Read the model definition and answer for the solid it produces. Units are mm, in the model's axes. A direction names the side the tool comes from. Round coordinates to 2 decimals unless told otherwise and drop trailing zeros. Order: outer loops, then holes, each group sorted by start corner. A loop starts at its lowest first (then second) coordinate and runs counter-clockwise, first axis right, second up. Notation, with made-up numbers: (-15, 56.25) - (24, 56.25) arc R17 cw to (24, 72.25) - close; hole circle Ø1 at (6, 22). An arc over 180 degrees is marked (long way). Answer as a JSON object with one key per item and string values. Group by question number.
Q1. A cutting plane is placed at A-A on y = 0. Determine the outline of the cut face in (x, z).
Q2. Given pin 1 Ø1 at (x, y) = (-5, -6) entering from +Z; pin 2 Ø1.5 at (y, z) = (-11.5, 0.5) entering from -X; pin 3 Ø8 at (x, y) = (-12.5, 7.5) entering from -Z; pin 4 Ø2 at (x, z) = (-24, 3.5) entering from +Y, each flat-ended and moving along its own axis, determine where each tip first touches the part or whether it passes through.
Q3. A tool of negligible diameter and unlimited length cuts with its end or side. For faces 5 (the flat face through (33.865, 16.365, 2.958)), 6 (the cylindrical face through (36.963, 15.287, 2.958)), 7 (the flat face through (24.6, 28.54, 2.96)), 8 (the flat face through (-28.476, -24.572, 2.958)), 9 (the flat face through (-31.105, 21.146, 2.958)), from which of +Z, -Z, +X, -X, +Y, -Y can it reach the whole face along a straight path? Write none if from no direction.
Q4. Consider line 1 (X direction, y = 32, z = 1.5); line 2 (X direction, y = 36, z = 0.75); line 3 (X direction, y = 18, z = 4.8). Determine where each line is inside the solid, lowest interval first.
Q5. The mould has two halves that part along Y. Classify faces 1 (the cylindrical face through (-36.963, -15.287, 2.958)), 2 (the flat face through (-24.572, 28.476, 2.958)), 3 (the flat face through (2.76, 37.51, 2.96)), 4 (the flat face through (16.365, -33.865, 2.958)): pulls with the +Y half, pulls with the -Y half, needs draft (parallel to the pull), parting line crosses it, or undercut.
```python
from build123d import *

# Parameters (mm, degrees)
SKETCH1_R           = 40
SKETCH1_R_2         = 10
BOSS_EXTRUDE1_DEPTH = 6
CUT_EXTRUDE1_START  = -6
CUT_EXTRUDE1_DEPTH  = 6
CIRPATTERN1_DEPTH   = 6


# Read off the part's stored shape, not the designer's step: CirPattern1
with BuildPart() as part:
    # Sketch1 → Boss-Extrude1 (new body)
    with BuildSketch(Plane.XY):
        Circle(SKETCH1_R)
        Circle(SKETCH1_R_2, mode=Mode.SUBTRACT)
    extrude(amount=BOSS_EXTRUDE1_DEPTH)

    # Sketch2 → Cut-Extrude1 (cut)
    with BuildSketch(Plane.XY.offset(6).offset(CUT_EXTRUDE1_START)):
        with BuildLine():
            Line((-3.690328017, 39.829404705), (-1.856322788, 35.255644098))
            ThreePointArc((-1.856322788, 35.255644098), (0, 34), (1.856322788, 35.255644098))
            Line((1.856322788, 35.255644098), (3.690328017, 39.829404705))
            ThreePointArc((3.690328017, 39.829404705), (0, 40), (-3.690328017, 39.829404705))
        make_face()
    extrude(amount=CUT_EXTRUDE1_DEPTH, mode=Mode.SUBTRACT)

    # CirPattern1 outline → CirPattern1 (cut)
    with BuildSketch(Plane.XY):
        with BuildLine():
            ThreePointArc((-10.917902263, 33.573885466), (-8.799847534, 32.841478094), (-7.331762018, 34.534788848))
            Line((-7.331762018, 34.534788848), (-6.744025354, 39.427377824))
            ThreePointArc((-6.744025354, 39.427377824), (-10.352761804, 38.637033052), (-13.873191632, 37.517123477))
            Line((-13.873191632, 37.517123477), (-10.917902263, 33.573885466))
        make_face()
        with BuildLine():
            Line((10.917902263, 33.573885466), (13.873191632, 37.517123477))
            ThreePointArc((13.873191632, 37.517123477), (10.352761804, 38.637033052), (6.744025354, 39.427377824))
            Line((6.744025354, 39.427377824), (7.331762018, 34.534788848))
            ThreePointArc((7.331762018, 34.534788848), (8.799847534, 32.841478094), (10.917902263, 33.573885466))
        make_face()
        with BuildLine():
            Line((19.235444741, 29.604122022), (23.110620163, 32.648112284))
            ThreePointArc((23.110620163, 32.648112284), (20, 34.641016152), (16.718784541, 36.338440301))
            Line((16.718784541, 36.338440301), (16.020199358, 31.46044481))
            ThreePointArc((16.020199358, 31.46044481), (17, 29.444863729), (19.235444741, 29.604122022))
        make_face()
        with BuildLine():
            Line((26.242123448, 23.616886586), (30.773098123, 25.554186192))
            ThreePointArc((30.773098123, 25.554186192), (28.284271248, 28.284271248), (25.554186192, 30.773098123))
            Line((25.554186192, 30.773098123), (23.616886586, 26.242123448))
            ThreePointArc((23.616886586, 26.242123448), (24.04163056, 24.04163056), (26.242123448, 23.616886586))
        make_face()
        with BuildLine():
            Line((31.46044481, 16.020199358), (36.338440301, 16.718784541))
            ThreePointArc((36.338440301, 16.718784541), (34.641016152, 20), (32.648112284, 23.110620163))
            Line((32.648112284, 23.110620163), (29.604122022, 19.235444741))
            ThreePointArc((29.604122022, 19.235444741), (29.444863729, 17), (31.46044481, 16.020199358))
        make_face()
        with BuildLine():
            Line((34.534788848, 7.331762018), (39.427377824, 6.744025354))
            ThreePointArc((39.427377824, 6.744025354), (38.637033052, 10.352761804), (37.517123477, 13.873191632))
            Line((37.517123477, 13.873191632), (33.573885466, 10.917902263))
            ThreePointArc((33.573885466, 10.917902263), (32.841478094, 8.799847534), (34.534788848, 7.331762018))
        make_face()
        with BuildLine():
            Line((35.255644098, -1.856322788), (39.829404705, -3.690328017))
            ThreePointArc((39.829404705, -3.690328017), (40, 0), (39.829404705, 3.690328017))
            Line((39.829404705, 3.690328017), (35.255644098, 1.856322788))
            ThreePointArc((35.255644098, 1.856322788), (34, 0), (35.255644098, -1.856322788))
        make_face()
        with BuildLine():
            Line((33.573885466, -10.917902263), (37.517123477, -13.873191632))
            ThreePointArc((37.517123477, -13.873191632), (38.637033052, -10.352761804), (39.427377823, -6.744025354))
            Line((39.427377823, -6.744025354), (34.534788848, -7.331762018))
            ThreePointArc((34.534788848, -7.331762018), (32.841478094, -8.799847534), (33.573885466, -10.917902263))
        make_face()
        with BuildLine():
            Line((29.604122022, -19.235444741), (32.648112283, -23.110620163))
            ThreePointArc((32.648112283, -23.110620163), (34.641016152, -20), (36.3384403, -16.718784541))
            Line((36.3384403, -16.718784541), (31.46044481, -16.020199358))
            ThreePointArc((31.46044481, -16.020199358), (29.444863729, -17), (29.604122022, -19.235444741))
        make_face()
        with BuildLine():
            Line((23.616886586, -26.242123448), (25.554186192, -30.773098123))
            ThreePointArc((25.554186192, -30.773098123), (28.284271247, -28.284271247), (30.773098123, -25.554186192))
            Line((30.773098123, -25.554186192), (26.242123448, -23.616886586))
            ThreePointArc((26.242123448, -23.616886586), (24.04163056, -24.04163056), (23.616886586, -26.242123448))
        make_face()
        with BuildLine():
            Line((16.020199358, -31.46044481), (16.718784541, -36.3384403))
            ThreePointArc((16.718784541, -36.3384403), (20, -34.641016151), (23.110620163, -32.648112283))
            Line((23.110620163, -32.648112283), (19.235444741, -29.604122022))
            ThreePointArc((19.235444741, -29.604122022), (17, -29.444863729), (16.020199358, -31.46044481))
        make_face()
        with BuildLine():
            Line((7.331762018, -34.534788848), (6.744025354, -39.427377823))
            ThreePointArc((6.744025354, -39.427377823), (10.352761804, -38.637033051), (13.873191632, -37.517123476))
            Line((13.873191632, -37.517123476), (10.917902263, -33.573885466))
            ThreePointArc((10.917902263, -33.573885466), (8.799847534, -32.841478094), (7.331762018, -34.534788848))
        make_face()
        with BuildLine():
            Line((-1.856322788, -35.255644098), (-3.690328017, -39.829404705))
            ThreePointArc((-3.690328017, -39.829404705), (0, -40), (3.690328017, -39.829404705))
            Line((3.690328017, -39.829404705), (1.856322788, -35.255644098))
            ThreePointArc((1.856322788, -35.255644098), (0, -34), (-1.856322788, -35.255644098))
        make_face()
        with BuildLine():
            Line((-10.917902263, -33.573885466), (-13.873191632, -37.517123476))
            ThreePointArc((-13.873191632, -37.517123476), (-10.352761804, -38.637033051), (-6.744025354, -39.427377823))
            Line((-6.744025354, -39.427377823), (-7.331762018, -34.534788848))
            ThreePointArc((-7.331762018, -34.534788848), (-8.799847534, -32.841478094), (-10.917902263, -33.573885466))
        make_face()
        with BuildLine():
            Line((-19.235444741, -29.604122022), (-23.110620163, -32.648112283))
            ThreePointArc((-23.110620163, -32.648112283), (-20, -34.641016151), (-16.718784541, -36.3384403))
            Line((-16.718784541, -36.3384403), (-16.020199358, -31.46044481))
            ThreePointArc((-16.020199358, -31.46044481), (-17, -29.444863729), (-19.235444741, -29.604122022))
        make_face()
        with BuildLine():
            Line((-26.242123448, -23.616886586), (-30.773098123, -25.554186192))
            ThreePointArc((-30.773098123, -25.554186192), (-28.284271247, -28.284271247), (-25.554186192, -30.773098123))
            Line((-25.554186192, -30.773098123), (-23.616886586, -26.242123448))
            ThreePointArc((-23.616886586, -26.242123448), (-24.04163056, -24.04163056), (-26.242123448, -23.616886586))
        make_face()
        with BuildLine():
            Line((-31.46044481, -16.020199358), (-36.3384403, -16.718784541))
            ThreePointArc((-36.3384403, -16.718784541), (-34.641016152, -20), (-32.648112283, -23.110620163))
            Line((-32.648112283, -23.110620163), (-29.604122022, -19.235444741))
            ThreePointArc((-29.604122022, -19.235444741), (-29.444863729, -17), (-31.46044481, -16.020199358))
        make_face()
        with BuildLine():
            Line((-34.534788848, -7.331762018), (-39.427377823, -6.744025354))
            ThreePointArc((-39.427377823, -6.744025354), (-38.637033052, -10.352761804), (-37.517123477, -13.873191632))
            Line((-37.517123477, -13.873191632), (-33.573885466, -10.917902263))
            ThreePointArc((-33.573885466, -10.917902263), (-32.841478094, -8.799847534), (-34.534788848, -7.331762018))
        make_face()
        with BuildLine():
            Line((-35.255644098, 1.856322788), (-39.829404705, 3.690328017))
            ThreePointArc((-39.829404705, 3.690328017), (-40, 0), (-39.829404705, -3.690328017))
            Line((-39.829404705, -3.690328017), (-35.255644098, -1.856322788))
            ThreePointArc((-35.255644098, -1.856322788), (-34, 0), (-35.255644098, 1.856322788))
        make_face()
        with BuildLine():
            Line((-33.573885466, 10.917902263), (-37.517123477, 13.873191632))
            ThreePointArc((-37.517123477, 13.873191632), (-38.637033052, 10.352761804), (-39.427377824, 6.744025354))
            Line((-39.427377824, 6.744025354), (-34.534788848, 7.331762018))
            ThreePointArc((-34.534788848, 7.331762018), (-32.841478094, 8.799847534), (-33.573885466, 10.917902263))
        make_face()
        with BuildLine():
            Line((-29.604122022, 19.235444741), (-32.648112284, 23.110620163))
            ThreePointArc((-32.648112284, 23.110620163), (-34.641016152, 20), (-36.338440301, 16.718784541))
            Line((-36.338440301, 16.718784541), (-31.46044481, 16.020199358))
            ThreePointArc((-31.46044481, 16.020199358), (-29.444863729, 17), (-29.604122022, 19.235444741))
        make_face()
        with BuildLine():
            Line((-23.616886586, 26.242123448), (-25.554186192, 30.773098123))
            ThreePointArc((-25.554186192, 30.773098123), (-28.284271248, 28.284271248), (-30.773098123, 25.554186192))
            Line((-30.773098123, 25.554186192), (-26.242123448, 23.616886586))
            ThreePointArc((-26.242123448, 23.616886586), (-24.04163056, 24.04163056), (-23.616886586, 26.242123448))
        make_face()
        with BuildLine():
            Line((-16.020199358, 31.46044481), (-16.718784541, 36.338440301))
            ThreePointArc((-16.718784541, 36.338440301), (-20, 34.641016152), (-23.110620163, 32.648112284))
            Line((-23.110620163, 32.648112284), (-19.235444741, 29.604122022))
            ThreePointArc((-19.235444741, 29.604122022), (-17, 29.444863729), (-16.020199358, 31.46044481))
        make_face()
    extrude(amount=CIRPATTERN1_DEPTH, mode=Mode.SUBTRACT)


solid = part.part
```
Result set:
{
 "1": {"outline": "(-34, 0) - (-10, 0) - (-10, 6) - (-34, 6) - close; (10, 0) - (34, 0) - (34, 6) - (10, 6) - close"},
 "2": {"pin 1": "passes through", "pin 2": "stops at x = -35.35", "pin 3": "stops at z = 0", "pin 4": "stops at y = 32.65"},
 "3": {"face 5": "+Z, -Z", "face 6": "+Z, -Z, +X, +Y", "face 7": "+Z, -Z, +X", "face 8": "+Z, -Z, -Y", "face 9": "+Z, -Z, -X"},
 "4": {"line 1": "x = -24 to -22.29, -16.1 to 16.1, 22.29 to 24", "line 2": "x = -16.67 to -12.74, -7.16 to -2.15, 2.15 to 7.16, 12.74 to 16.67", "line 3": "x = -29.18 to 29.18"},
 "5": {"face 1": "pulls with the -Y half", "face 2": "undercut", "face 3": "pulls with the +Y half", "face 4": "undercut"}
}
